Geometry: final body of the model. Coordinates: model frame, mm. Face numbers are marked on the shaded views. A direction names the side the tool comes from. Coordinates: 2 decimals unless noted, no trailing zeros. Write each loop counter-clockwise with the first axis right and the second up, starting at its lowest first coordinate (ties: lowest second). Pieces come first, ordered by that corner, then holes. Notation, with made-up numbers: (64.25, 76.5) -> (79.25, 76.5) arc R22 cw to (79.25, 90.5) -> close; hole circle Ø8 at (-28, 79). An arc over 180 degrees is marked (long way). One line per item, written item: value.
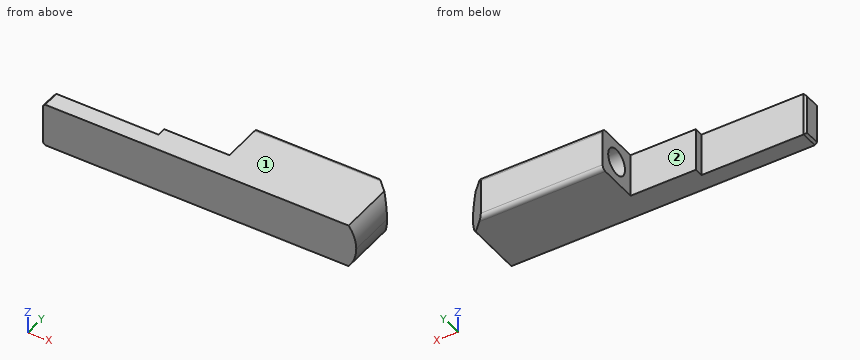
```python
from build123d import *

# Parameters (mm, degrees)
F0_W      = 72
F0_H      = 16
F1_DEPTH  = 10
F2_SIZE   = 5
F4_DEPTH  = 10
F5_SIZE   = 0.5
F6_R      = 1
F8_DEPTH  = 25
F10_D     = 6
F10_DEPTH = 10
F10_TIP   = 1.8025818571


with BuildPart() as f1:
    # F0 (on Top) → F1 (new body)
    with BuildSketch(Plane.XY):
        Rectangle(F0_W, F0_H)
    extrude(amount=F1_DEPTH)

    # F2
    f2_edges = [f1.edges().sort_by_distance(p)[0] for p in [
        (36, 8, 5),
    ]]
    chamfer(f2_edges, length=F2_SIZE)

    # F3 (on face) → F4 (cut, through all)
    with BuildSketch(Plane.XY.offset(10)):
        Polygon((3, -2), (3, 8), (-36, 8), (-36, -4), (-12, -4), (-12, -2), align=None)
    extrude(amount=-F4_DEPTH, mode=Mode.SUBTRACT)

    # F5
    f5_edges = [f1.edges().sort_by_distance(p)[0] for p in [
        (-36, -4, 5),
        (-36, -6, 10),
        (-36, -6, 0),
    ]]
    chamfer(f5_edges, length=F5_SIZE)

    # F6
    f6_edges = [f1.edges().sort_by_distance(p)[0] for p in [
        (17, 8, 10),
        (17, 8, 0),
    ]]
    fillet(f6_edges, radius=F6_R)

    # F7 (on face) → F8 (cut)
    with BuildSketch(Plane(origin=(0, 8, 0), x_dir=(-1, 0, 0), z_dir=(0, 1, 0))):
        with BuildLine():
            ThreePointArc((-34.2449979984, 0), (-35.5485092564, 2.3504702292), (-36, 5))
            Line((-36, 5), (-36, 0))
            Line((-36, 0), (-34.2449979984, 0))
        make_face()
        with BuildLine():
            ThreePointArc((-36, 5), (-35.5485092564, 7.6495297708), (-34.2449979984, 10))
            Line((-34.2449979984, 10), (-36, 10))
            Line((-36, 10), (-36, 5))
        make_face()
    extrude(amount=-F8_DEPTH, mode=Mode.SUBTRACT)

    # F10
    with Locations(Plane(origin=(3, 0, 0), x_dir=(0, -1, 0), z_dir=(-1, 0, 0))):
        with Locations((-3, 5)):
            Hole(F10_D / 2, depth=F10_DEPTH)
            with Locations((0, 0, -(F10_DEPTH + F10_TIP / 2))):  # 118° drill point
                Cone(0, F10_D / 2, F10_TIP, mode=Mode.SUBTRACT)


solid = f1.part
```
(1) Line query: line 1 (Z direction, x = 9.5, y = 3); line 2 (Y direction, x = 11.25, z = 5); line 3 (Y direction, x = -17.5, z = 9.25). Output: solid intervals per line, ascending. Write a range as [from, to].
Responses:
line 1: z = [0, 2], [8, 10]
line 2: y = [-8, 0], [6, 8]
line 3: y = [-8, -4]
(2) Reachability of the marked faces 1 and 2 from +Z, -Z, +X, -X, +Y, -Y: full face, straight path, thin tool, end or side. Return the list, or none.
Responses:
face 1: +Z, +X, -X, +Y, -Y
face 2: +Z, -Z, -X, +Y
(3) Section A-A (x = 4). Return the cut outline in (y, z), then the cut area to 3 significant figures.
Responses:
outline: (-8, 0) -> (7, 0) arc R1 ccw to (8, 1) -> (8, 9) arc R1 ccw to (7, 10) -> (-8, 10) -> close; hole circle Ø6 at (3, 5)
area: 131 mm2
(4) Section C-C (x = -27). Return the cut outline in (y, z), then the cut area to 3 significant figures.
Responses:
outline: (-8, 0) -> (-4, 0) -> (-4, 10) -> (-8, 10) -> close
area: 40.0 mm2
(5) First-contact query: pin 1 (3 mm diameter, centred on y = 1, z = 7, fed in from -X); pin 2 (0.6 mm diameter, centred on y = -2.5, z = 5, fed in from -X); pin 3 (2 mm diameter, centred on y = -2.5, z = 8, fed in from +X); pin 4 (3 mm diameter, centred on y = 1.5, z = 6.5, fed in from +X). Flat tips, straight axial feed; report the tip coordinate or a pass-through.
Responses:
pin 1: stops at x = 3
pin 2: stops at x = -12
pin 3: stops at x = 35.75
pin 4: stops at x = 36
(6) Section B-B (y = -0.75). Return the cut outline in (x, z) (3 decimals), then the cut area to 3 significant figures.
Responses:
outline: (3, 0) -> (34.245, 0) arc R8 ccw to (34.245, 10) -> (3, 10) -> close
area: 324 mm2
